Input: part model. Units: mm. Frame: model coordinates. A direction names the side the tool comes from. Coordinates: 2 decimals unless noted, no trailing zeros. Write each loop counter-clockwise with the first axis right and the second up, starting at its lowest first coordinate (ties: lowest second). Pieces come first, ordered by that corner, then holes. Notation, with made-up numbers: (44, -26) - (85, -26) arc R22 ccw to (85, 12) - close; hole circle Ø2 at (-21, 56). An arc over 180 degrees is marked (long way). Put each result on its own line as item: value. Start each with the question number.
1. Cut plane C-C, the plane x = -2.5. Return loops of the section in (y, z).
2. Pull-direction query (Z, two-part tool) for faces 1 (the cylindrical face through (0, 0, -24)), 2 (the flat face through (-10, 11, -1)); classes: released by +Z, released by -Z, zero draft, split by the parting line, or undercut.
3. Cut plane A-A, the plane y = 0. Return loops of the section in (x, z), and give its area (3 significant figures).
4. Cut plane D-D, the plane y = 35. Count the separate pieces of the cut face and the enclosed holes in it, and give its area (3 significant figures).
5. Pin query (flat end, axial travel): pin 1 (6 mm diameter, centred on x = 1.5, z = -40, fed in from +Y); pin 2 (2 mm diameter, centred on x = -2.5, z = -20.5, fed in from +Y); pin 3 (4 mm diameter, centred on y = 34, z = -49.5, fed in from +X); pin 4 (7 mm diameter, centred on y = 0, z = 0, fed in from +X). Return the tip coordinate at first contact, or that it passes through.
6. Cut plane B-B, the plane x = 4.75. Return loops of the section in (y, z).
7. Line query: line 1 (Z direction, x = -0.5, y = 0); line 2 (Y direction, x = 6.75, z = 32); line 3 (Z direction, x = 5.25, y = 0). Output: solid intervals per line, ascending.
8. Access query for faces 3 (the flat face through (10, -1, -11)), 4 (the flat face through (0, 6, 33)). Directions: +Z, -Z, +X, -X, +Y, -Y. A direction counts if a zero-diameter tool reaches every point of the face in a straight line with its end or side. Return the directions, or none.
from build123d import *

# Parameters (mm, degrees)
F3_DEPTH = 25


with BuildPart() as f1:
    # F0 (on Front) → F1 (revolve)
    with BuildSketch(Plane.XZ):
        with BuildLine():
            Line((-10, 55), (-10, 4))
            Line((-10, 4), (10, 4))
            Line((10, 4), (10, 55))
            ThreePointArc((10, 55), (0, 45), (-10, 55))
        make_face()
        with BuildLine():
            ThreePointArc((10, 55), (0, 65), (-10, 55))
            ThreePointArc((-10, 55), (0, 45), (10, 55))
        make_face()
    revolve(axis=Axis((-12.7272796474, 0, 0), (1, 0, 0)))

    # F2 (on face) → F3 (cut)
    with BuildSketch(Plane(origin=(-10, 0, 0), x_dir=(0, -1, 0), z_dir=(-1, 0, 0))):
        with BuildLine():
            Line((-30.4750671187, -31.7375217071), (-18.5129969259, -15.2731445623))
            ThreePointArc((-18.5129969259, -15.2731445623), (-22.8253563911, -7.416407865), (-23.9546582597, 1.4745669397))
            Line((-23.9546582597, 1.4745669397), (-43.3096944075, 7.7633994054))
            ThreePointArc((-43.3096944075, 7.7633994054), (-41.846486717, -13.5967477525), (-30.4750671187, -31.7375217071))
        make_face()
        with BuildLine():
            Line((20.7668631862, -38.7909447346), (8.8047929934, -22.3265675898))
            ThreePointArc((8.8047929934, -22.3265675898), (0, -24), (-8.8047929934, -22.3265675898))
            Line((-8.8047929934, -22.3265675898), (-20.7668631862, -38.7909447346))
            ThreePointArc((-20.7668631862, -38.7909447346), (0, -44), (20.7668631862, -38.7909447346))
        make_face()
        with BuildLine():
            ThreePointArc((23.9546582597, 1.4745669397), (23.9886618867, 0.7376319429), (24, 0))
            ThreePointArc((24, 0), (22.5866323986, -8.1144338613), (18.5129969259, -15.2731445623))
            Line((18.5129969259, -15.2731445623), (30.4750671187, -31.7375217071))
            ThreePointArc((30.4750671187, -31.7375217071), (40.4777899176, -17.2495948761), (44, 0))
            ThreePointArc((44, 0), (43.8270838291, 3.8970146311), (43.3096944075, 7.7633994054))
            Line((43.3096944075, 7.7633994054), (23.9546582597, 1.4745669397))
        make_face()
        with BuildLine():
            ThreePointArc((-20.2464543272, 12.8872451352), (-14.106846055, 19.416407865), (-6, 23.2379000772))
            Line((-6, 23.2379000772), (-6, 43.5889894354))
            ThreePointArc((-6, 43.5889894354), (-25.8625511009, 35.5967477525), (-39.601490475, 19.1760776009))
            Line((-39.601490475, 19.1760776009), (-20.2464543272, 12.8872451352))
        make_face()
        with BuildLine():
            ThreePointArc((6, 23.2379000772), (14.106846055, 19.416407865), (20.2464543272, 12.8872451352))
            Line((20.2464543272, 12.8872451352), (39.601490475, 19.1760776009))
            ThreePointArc((39.601490475, 19.1760776009), (25.8625511009, 35.5967477525), (6, 43.5889894354))
            Line((6, 43.5889894354), (6, 23.2379000772))
        make_face()
    extrude(amount=-F3_DEPTH, mode=Mode.SUBTRACT)


solid = f1.part
Report:
1. outline: circle Ø129.36 at (0, 0); hole (-43.31, 7.76) arc R44 ccw to (-30.48, -31.74) - (-18.51, -15.27) arc R24 cw to (-23.95, 1.47) - close; hole (-39.6, 19.18) - (-20.25, 12.89) arc R24 cw to (-6, 23.24) - (-6, 43.59) arc R44 ccw to start; hole (-20.77, -38.79) arc R44 ccw to (20.77, -38.79) - (8.8, -22.33) arc R24 cw to (-8.8, -22.33) - close; hole circle Ø8 at (0, 0); hole (6, 23.24) arc R24 cw to (20.25, 12.89) - (39.6, 19.18) arc R44 ccw to (6, 43.59) - close; hole (18.51, -15.27) - (30.48, -31.74) arc R44 ccw to (43.31, 7.76) - (23.95, 1.47) arc R24 cw to start
2. face 1: undercut
2. face 2: zero draft
3. outline: (-10, -55) arc R10 ccw to (10, -55) - (10, -44) - (-10, -44) - close; (-10, -24) - (10, -24) - (10, -4) - (-10, -4) - close; (-10, 4) - (10, 4) - (10, 55) arc R10 ccw to (-10, 55) - close
3. area: 1,950 mm^2
4. separate pieces: 3
4. enclosed holes: 0
4. area: 1,270 mm^2
5. pin 1: stops at y = 53.35
5. pin 2: stops at y = 61.75
5. pin 3: stops at x = 9.52
5. pin 4: passes through
6. outline: circle Ø127.6 at (0, 0); hole (-43.31, 7.76) arc R44 ccw to (-30.48, -31.74) - (-18.51, -15.27) arc R24 cw to (-23.95, 1.47) - close; hole (-39.6, 19.18) - (-20.25, 12.89) arc R24 cw to (-6, 23.24) - (-6, 43.59) arc R44 ccw to start; hole (-20.77, -38.79) arc R44 ccw to (20.77, -38.79) - (8.8, -22.33) arc R24 cw to (-8.8, -22.33) - close; hole circle Ø8 at (0, 0); hole (6, 23.24) arc R24 cw to (20.25, 12.89) - (39.6, 19.18) arc R44 ccw to (6, 43.59) - close; hole (18.51, -15.27) - (30.48, -31.74) arc R44 ccw to (43.31, 7.76) - (23.95, 1.47) arc R24 cw to start
7. line 1: z = -64.99 to -44, -24 to -4, 4 to 64.99
7. line 2: y = -53.54 to -30.2, -6 to 6, 30.2 to 53.54
7. line 3: z = -63.51 to -44, -24 to -4, 4 to 63.51
8. face 3: +Z, -Z, +X, +Y, -Y
8. face 4: +X, -X
